from build123d import *

# Parameters (mm, degrees)
SKETCH1_W           = 30
SKETCH1_H           = 30
BOSS_EXTRUDE1_DEPTH = 6
SKETCH2_W           = 6
SKETCH2_H           = 30
BOSS_EXTRUDE2_DEPTH = 30
SKETCH3_R           = 3
CUT_EXTRUDE1_DEPTH  = 46.793012567


with BuildPart() as part:
    # Sketch1 → Boss-Extrude1 (new body)
    with BuildSketch(Plane.XY):
        Rectangle(SKETCH1_W, SKETCH1_H)
    extrude(amount=BOSS_EXTRUDE1_DEPTH)

    # Sketch2 → Boss-Extrude2 (add)
    with BuildSketch(Plane.XY.offset(6)):
        with Locations((-12, 0)):
            Rectangle(SKETCH2_W, SKETCH2_H)
    extrude(amount=BOSS_EXTRUDE2_DEPTH)

    # Sketch3 → Cut-Extrude1 (cut, through all)
    with BuildSketch(Plane(origin=(-9, 0, 0), x_dir=(0, 0, -1), z_dir=(1, 0, 0))):
        with Locations((-21, 0)):
            Circle(SKETCH3_R)
    extrude(amount=-CUT_EXTRUDE1_DEPTH, mode=Mode.SUBTRACT)


solid = part.part
Work out the finished part from the listing and answer in its coordinate system (mm). A direction names the side the tool comes from. Coordinates: 2 decimals unless noted, no trailing zeros. Loops run counter-clockwise (first coordinate to the right, second up) from the corner with the lowest first, then second, coordinate; pieces in that order, holes last. Notation, with made-up numbers: M 31.25,59.5 L 66.25,59.5 A15 ccw 66.25,75.5 Z; hole C 70.5,-23.5 d3. An arc over 180 degrees is marked long. Answer in a Markdown table with one row per item. Add a question column.
1. Find section B-B, the plane z = 21. Write down the section's boundary in (x, y).
2. Find section C-C, the plane y = 12.5. Write down the section's boundary in (x, z).
3. The mould has two halves that part along Z. Classify faces 1 (the flat face through (3, 0, 6)), 2 (the cylindrical face through (-12, 0, 24)), 3 (the flat face through (15, 0, 3)): pulls with the +Z half, pulls with the -Z half, needs draft (parallel to the pull), parting line crosses it, or undercut.
4. A flat-ended cylindrical pin translates along its axis: P1, Ø12, axis at x = 8.5, y = 0.5, coming from the +Z side. Find the tip coordinate at first contact, or state that the pin passes through.
5. Find section D-D, the plane x = 10. Write down the section's boundary in (y, z).
6. Consider L1, parallel to Y at x = -11.55, z = 21; L2, parallel to Z at x = 13.5, y = -5.25; L3, parallel to X at y = 13.25, z = 21. Determine where each line is inside the solid, lowest interval first.
7. Find section A-A, the plane y = 0. Write down the section's boundary in (x, z).
8. A tool of negligible diameter and unlimited length cuts with its end or side. For faces 4 (the flat face through (-10, 15, 10)), 5 (the flat face through (-9, 0, 17)), from which of +Z, -Z, +X, -X, +Y, -Y can it reach the whole face along a straight path? Write none if from no direction.
Reported:
| question | item | result |
|---|---|---|
| 1 | outline | M -15,-15 L -9,-15 L -9,-3 L -15,-3 Z; M -15,3 L -9,3 L -9,15 L -15,15 Z |
| 2 | outline | M -15,0 L 15,0 L 15,6 L -9,6 L -9,36 L -15,36 Z |
| 3 | face 1 | pulls with the +Z half |
| 3 | face 2 | undercut |
| 3 | face 3 | needs draft |
| 4 | P1 | stops at z = 6 |
| 5 | outline | M -15,0 L 15,0 L 15,6 L -15,6 Z |
| 6 | L1 | y = -15 to -3, 3 to 15 |
| 6 | L2 | z = 0 to 6 |
| 6 | L3 | x = -15 to -9 |
| 7 | outline | M -15,0 L 15,0 L 15,6 L -9,6 L -9,18 L -15,18 Z; M -15,24 L -9,24 L -9,36 L -15,36 Z |
| 8 | face 4 | +Z, -Z, +X, -X, +Y |
| 8 | face 5 | +Z, +X, +Y, -Y |
